Work out the finished part from the listing and answer in its coordinate system (mm). Round coordinates to 2 decimals unless told otherwise and drop trailing zeros. Write each loop counter-clockwise with the first axis right and the second up, starting at its lowest first coordinate (ties: lowest second). Pieces come first, ordered by that corner, then holes. Notation, with made-up numbers: (-38.5, 13.25) -> (-20.5, 13.25) arc R18 ccw to (-20.5, 24.25) -> close; hole circle Ø3 at (69.25, -16). An arc over 180 degrees is marked (long way). Answer as a JSON object with one key per item and string values. Group by question number.
Autodesk Inventor part; units mm, degrees
ref_plane "YZ Plane" through (0, 0, 0) normal (1, 0, 0) x (0, 1, 0)
ref_plane "XZ Plane" through (0, 0, 0) normal (0, 1, 0) x (-1, 0, 0)
ref_plane "XY Plane" through (0, 0, 0) normal (0, 0, 1) x (1, 0, 0)
sketch "Sketch1" plane through (0, 0, 0) normal (0, 0, 1) x (1, 0, 0)
  line L0 (0, 0) -> (1320.8, 0)
  line L1 (1320.8, 0) -> (1320.8, 76.2)
  line L2 (1320.8, 76.2) -> (0, 76.2)
  line L3 (0, 76.2) -> (0, 0)
  line L4 (1193.8, 0) -> (1320.8, 6.6558)
  line L5 (0, 76.2) -> (191.0937, 0)
  dimension "d0" = 76.2
  dimension "d1" = 1320.8
  dimension "d2" = 3
  dimension "d3" = 127
  dimension "d5" = 21.74
extrude "Extrusion1" add sketch "Sketch1" along normal blind 11.938 contours L5 L2 L1 L4 L0
properties part number "Antitorque span" material "Wood (Oak)"
1) Straight lines are drawn through the part: L1, parallel to Y at x = 109.5, z = 6.25; L2, parallel to Y at x = 53, z = 3.5. For each, find the intervals that lie inside material, in ascending order.
2) A cutting plane is placed at A-A on z = 3.5. Determine the outline of the cut face in (x, y), plus the area to 3 significant figures.
3) A cutting plane is placed at B-B on y = 25.5. Determine the outline of the cut face in (x, z).
4) A cutting plane is placed at C-C on x = 96. Determine the outline of the cut face in (y, z), plus the area to 3 significant figures.
Established:
{
 "1": {"L1": "y = 32.54 to 76.2", "L2": "y = 55.07 to 76.2"},
 "2": {"outline": "(0, 76.2) -> (191.09, 0) -> (1193.8, 0) -> (1320.8, 6.66) -> (1320.8, 76.2) -> close", "area": "92,900 mm²"},
 "3": {"outline": "(127.15, 0) -> (1320.8, 0) -> (1320.8, 11.94) -> (127.15, 11.94) -> close"},
 "4": {"outline": "(37.92, 0) -> (76.2, 0) -> (76.2, 11.94) -> (37.92, 11.94) -> close", "area": "457 mm²"}
}
